Design review of the part shown in the three views and the two pictorial views. Dimensions are in mm from the part's minimum x, y and z. A direction names the side the tool comes from. Coordinates: 2 decimals unless noted, no trailing zeros. Write each loop counter-clockwise with the first axis right and the second up, starting at its lowest first coordinate (ties: lowest second). Pieces come first, ordered by that corner, then holes. Notation, with made-up numbers: M 74,41 L 118,41 A17 ccw 118,46 Z; hole C -3,60 d3. An arc over 180 degrees is marked long. Answer as a JSON object with one key per item and string values.
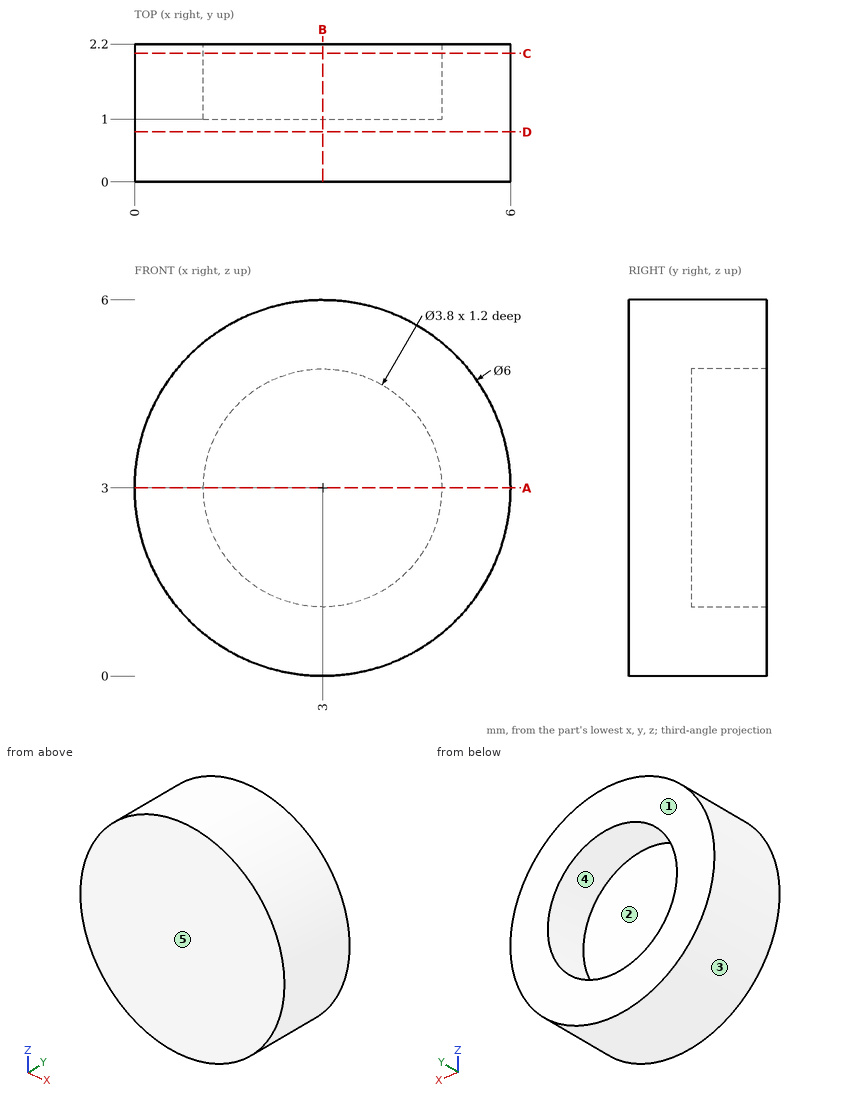
(1) Draft analysis for pull direction Z (two halves, no side actions). For the marked faces 3, 4 and 5, state which applies: released by +Z, released by -Z, zero draft, split by the parting line, or undercut.
Results list:
{"face 3": "split by the parting line", "face 4": "undercut", "face 5": "zero draft"}
(2) Add section C-C on y = 2.05. Give the boundary of the cut face in (x, z).
Results list:
{"outline": "C 3,3 d6; hole C 3,3 d3.8"}
(3) Add section B-B on x = 3. Give the boundary of the cut face in (y, z).
Results list:
{"outline": "M 0,0 L 2.2,0 L 2.2,1.1 L 1,1.1 L 1,4.9 L 2.2,4.9 L 2.2,6 L 0,6 Z"}
(4) For pin 1 Ø1 at (x, y) = (4, 2) entering from -Z; pin 2 Ø2.5 at (x, z) = (3, 3) entering from +Y, all flat-tipped, find the tip position at first contact; note any pin that passes through.
Results list:
{"pin 1": "z = 0.04", "pin 2": "y = 1"}
(5) Add section D-D on y = 0.8. Give the boundary of the cut face in (x, z), and give its area (3 significant figures).
Results list:
{"outline": "C 3,3 d6", "area": "28.3 mm²"}
(6) Add section A-A on z = 3. Give the boundary of the cut face in (x, y).
Results list:
{"outline": "M 0,0 L 6,0 L 6,2.2 L 4.9,2.2 L 4.9,1 L 1.1,1 L 1.1,2.2 L 0,2.2 Z"}
(7) For the marked faces 1 and 2, list the 3-axis set-ups (+Z, -Z, +X, -X, +Y, -Y) from which the entire face can be reached by the end or side of a thin tool; tool diameter is ignored.
Results list:
{"face 1": "+Z, -Z, +X, -X, +Y", "face 2": "+Y"}
(8) Wall thickness on line 1 along Z through (x, y) = (3, 1.7); line 2 along Z through (x, y) = (4.1, 1.6): over which ranges is each line inside the solid? List them lowest first. Write a range as from..to.
Results list:
{"line 1": "0..1.1, 4.9..6", "line 2": "0.21..1.45, 4.55..5.79"}
